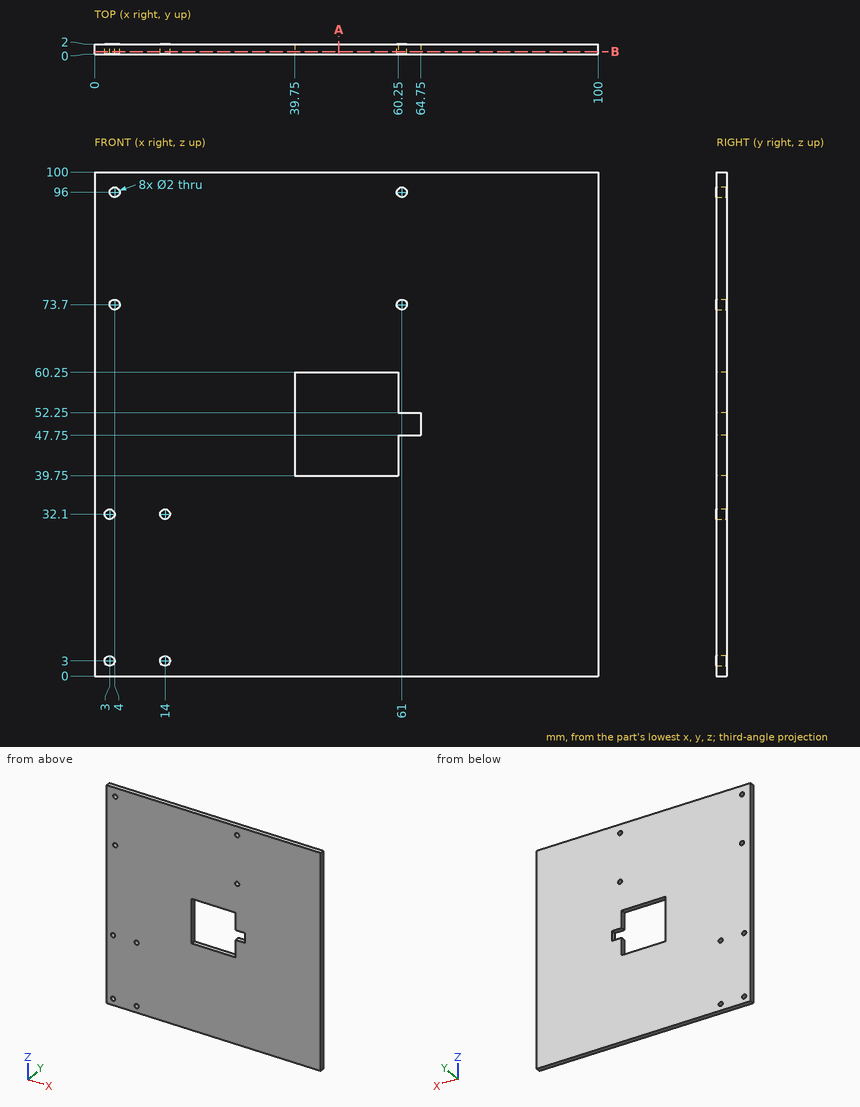
Job drawing, mm, ordinate dimensions from the low corner. One solid piece. Round coordinates to 2 decimals unless told otherwise and drop trailing zeros. Order: outer loops, then holes, each group sorted by start corner. A loop starts at its lowest first (then second) coordinate and runs counter-clockwise, first axis right, second up. Notation, with made-up numbers: (-11, 83.5) -> (36, 83.5) arc R25 ccw to (36, 116.5) -> close; hole circle Ø9 at (-3.5, 5.25). An arc over 180 degrees is marked (long way). Answer in a Markdown table with one row per item.
1) Band-saw the part on A-A on x = 48.5. Give the cut face in (y, z), and give its area (3 significant figures).
Values:
| item | result |
|---|---|
| outline | (0, 0) -> (2, 0) -> (2, 39.75) -> (0, 39.75) -> close; (0, 60.25) -> (2, 60.25) -> (2, 100) -> (0, 100) -> close |
| area | 159 mm2 |
2) Wall check: L1, parallel to X at y = 1.5, z = 32.1; L2, parallel to X at y = 0.9, z = 96; L3, parallel to Z at x = 61, y = 1.35. Give the ranges that are in metal, low to high.
Values:
| item | result |
|---|---|
| L1 | 0 to 2, 4 to 13, 15 to 100 |
| L2 | 0 to 3, 5 to 60, 62 to 100 |
| L3 | 0 to 47.75, 52.25 to 72.7, 74.7 to 95, 97 to 100 |
3) Band-saw the part on B-B on y = 0.5. Give the number of separate pieces and of enclosed holes in the cut face, and give its area (3 significant figures).
Values:
| item | result |
|---|---|
| separate pieces | 1 |
| enclosed holes | 9 |
| area | 9,530 mm2 |
